from build123d import *

# Parameters (mm, degrees)
D_GAGEMENT_M2_51_D           = 2.7
R_P_TITION_CIRCULAIRE1_COUNT = 4
ENL_V_MAT_EXTRU_1_DEPTH      = 52.894616773


with BuildPart() as part:
    # Esquisse1 → Révolution1 (revolve)
    with BuildSketch(Plane.XY, mode=Mode.PRIVATE) as r_volution1_sk:
        with BuildLine():
            Line((-11.382864376, 0), (-3, 0))
            Line((-3, 0), (-3, 2))
            Line((-3, 2), (-5, 2))
            Line((-5, 2), (-5, 3))
            Line((-5, 3), (-6, 3))
            Line((-6, 3), (-6, 5.648095238))
            ThreePointArc((-6, 5.648095238), (-6.091117155, 5.935870879), (-6.331259276, 6.118761328))
            Line((-6.331259276, 6.118761328), (-25.034076062, 12.823996539))
            ThreePointArc((-25.034076062, 12.823996539), (-25.532706049, 12.955671634), (-26.046520404, 13))
            Line((-26.046520404, 13), (-35.525, 13))
            Line((-35.525, 13), (-35.525, 10))
            Line((-35.525, 10), (-26.767640687, 10))
            ThreePointArc((-26.767640687, 10), (-25.61959039, 9.771638598), (-24.646320344, 9.121320344))
            Line((-24.646320344, 9.121320344), (-18.453932188, 2.928932188))
            ThreePointArc((-18.453932188, 2.928932188), (-15.2096987, 0.761204675), (-11.382864376, 0))
        make_face()
    revolve(r_volution1_sk.sketch.rotate(Axis((0, 5.07757265, 0), (0, -1, 0)), 270), axis=Axis((0, 5.07757265, 0), (0, -1, 0)))

    # Dégagement M2.51 (through all)
    with Locations(Plane(origin=(0, 13, 0), x_dir=(1, 0, 0), z_dir=(0, 1, 0))):
        with Locations((-32.525, 0)):
            d_gagement_m2_51 = Hole(D_GAGEMENT_M2_51_D / 2)

    # Répétition circulaire1: Dégagement M2.51 ×4 about axis
    r_p_tition_circulaire1_axis = Axis((0, 0, 0), (0, 1, 0))
    for i in range(1, R_P_TITION_CIRCULAIRE1_COUNT):
        add(d_gagement_m2_51.rotate(r_p_tition_circulaire1_axis, i * 360 / R_P_TITION_CIRCULAIRE1_COUNT), mode=Mode.SUBTRACT)

    # Esquisse4 → Enlèv. mat.-Extru.1 (cut, through all)
    with BuildSketch(Plane(origin=(0, 13, 0), x_dir=(1, 0, 0), z_dir=(0, 1, 0))):
        with BuildLine():
            ThreePointArc((3e-09, 35.525), (2.121320345, 34.646320343), (3, 32.525))
            Line((3, 32.525), (3, 13))
            ThreePointArc((3, 13), (5.928932188, 5.928932188), (13, 3))
            Line((13, 3), (32.525, 3))
            ThreePointArc((32.525, 3), (34.646320344, 2.121320344), (35.525, 0))
            ThreePointArc((35.525, 0), (25.119968403, 25.119968401), (3e-09, 35.525))
        make_face()
        with BuildLine():
            ThreePointArc((-3, 32.525), (-2.121320343, 34.646320345), (3e-09, 35.525))
            ThreePointArc((3e-09, 35.525), (-25.119968401, 25.119968403), (-35.525, 0))
            ThreePointArc((-35.525, 0), (-34.646320344, 2.121320344), (-32.525, 3))
            Line((-32.525, 3), (-13, 3))
            ThreePointArc((-13, 3), (-5.928932188, 5.928932188), (-3, 13))
            Line((-3, 13), (-3, 32.525))
        make_face()
        with BuildLine():
            ThreePointArc((0, -35.525), (25.119968402, -25.119968402), (35.525, 0))
            ThreePointArc((35.525, 0), (34.646320344, -2.121320344), (32.525, -3))
            Line((32.525, -3), (13, -3))
            ThreePointArc((13, -3), (5.928932188, -5.928932188), (3, -13))
            Line((3, -13), (3, -32.525))
            ThreePointArc((3, -32.525), (2.121320344, -34.646320344), (0, -35.525))
        make_face()
        with BuildLine():
            ThreePointArc((-32.525, -3), (-34.646320344, -2.121320344), (-35.525, 0))
            ThreePointArc((-35.525, 0), (-25.119968402, -25.119968402), (0, -35.525))
            ThreePointArc((0, -35.525), (-2.121320344, -34.646320344), (-3, -32.525))
            Line((-3, -32.525), (-3, -13))
            ThreePointArc((-3, -13), (-5.928932188, -5.928932188), (-13, -3))
            Line((-13, -3), (-32.525, -3))
        make_face()
    extrude(amount=-ENL_V_MAT_EXTRU_1_DEPTH, mode=Mode.SUBTRACT)


solid = part.part
Can you work these out from the model? Positions are in its coordinate system, mm. A direction names the side the tool comes from. Coordinates: 2 decimals unless noted, no trailing zeros. Write each loop counter-clockwise with the first axis right and the second up, starting at its lowest first coordinate (ties: lowest second). Pieces come first, ordered by that corner, then holes. Notation, with made-up numbers: (-15, 72) - (35, 72) arc R27 cw to (35, 102) - close; hole circle Ø2 at (30.5, 33). An arc over 180 degrees is marked (long way). Return JSON: item names as keys, results as strings. Group by question number.
Item 1: We'd pull the mould along X, two halves only. Please class faces 5 (the face through (-0.68, 6.26, 6.69)), 6 (the face through (3, 8, 20)), 7 (the face through (-0.049, 5.982, -21.507)), 8 (the face through (-20, 8, 3)): pulls with the +X half, pulls with the -X half, needs draft (parallel to the pull), parting line crosses it, or undercut.
Item 2: I'm going to push flat-ended pins straight in: pin 1 Ø4 at (y, z) = (11, -3.5) entering from +X; pin 2 Ø8 at (x, z) = (-25.5, 6) entering from -Y; pin 3 Ø6.5 at (x, y) = (20, 7.5) entering from -Z. Where does each tip first touch, or does it pass through?
Item 3: Which directions (+Z, -Z, +X, -X, +Y, -Y) give clear straight access to the entire face, cutting with the end or side of a thin tool? Please do faces 1 (the face through (-31, 10, 0)), 2 (the face through (-21, 8, -3)), 3 (the face through (3, 8, -21)), 4 (the face through (4.88, 2.51, -1.08)).
Item 4: If we section it at B-B (y = 4.5): Write out the boundary of the cut face in (x, z) (3 decimals), then the cut area to 3 significant figures.
Item 5: Please list where these lines run through material, in increasing order: probe 1 along X at (y, z) = (10.5, 29); probe 2 along Z at (x, y) = (11, 6).
Item 6: If we section it at A-A (y = 11.25): Count the separate pieces of the cut face and the enclosed holes in it, then the cut area to 3 significant figures.
Return value:
{
 "1": {"face 5": "undercut", "face 6": "pulls with the +X half", "face 7": "parting line crosses it", "face 8": "needs draft"},
 "2": {"pin 1": "stops at x = 35.12", "pin 2": "stops at y = 7.53", "pin 3": "stops at z = -3"},
 "3": {"face 1": "+Z, -Z, -X, -Y", "face 2": "-Z, -X, +Y, -Y", "face 3": "-Z, +X, +Y, -Y", "face 4": "+Y"},
 "4": {"outline": "(-19.799, -3) - (-13, -3) arc R10 cw to (-3, -13) - (-3, -19.799) arc R20.025 ccw to (3, -19.799) - (3, -13) arc R10 cw to (13, -3) - (19.799, -3) arc R20.025 ccw to (19.799, 3) - (13, 3) arc R10 cw to (3, 13) - (3, 19.799) arc R20.025 ccw to (-3, 19.799) - (-3, 13) arc R10 cw to (-13, 3) - (-19.799, 3) arc R20.025 ccw to start; hole circle Ø12 at (0, 0)", "area": "416 mm^2"},
 "5": {"probe 1": "x = -3 to 3", "probe 2": "z = -3.2 to 3.2"},
 "6": {"separate pieces": "4", "enclosed holes": "4", "area": "321 mm^2"}
}
